Input: part model. Units: mm. Frame: model coordinates. A direction names the side the tool comes from. Give positions to 0.01 mm unless a question says otherwise; leave off trailing zeros. Order: outer loops, then holes, each group sorted by start corner. A loop starts at its lowest first (then second) coordinate and runs counter-clockwise, first axis right, second up. Notation, with made-up numbers: (-8.75, 57.25) - (7.25, 57.25) arc R23 cw to (7.25, 87.25) - close; hole circle Ø7 at (-5, 84.25). An arc over 180 degrees is marked (long way). Use a Markdown table: item, result.
from build123d import *

# Parameters (mm, degrees)
F0_W     = 19.05
F0_H     = 3.175
F1_DEPTH = 2.54


with BuildPart() as f1:
    # F0 (on Front) → F1 (new body)
    with BuildSketch(Plane.XZ):
        with BuildLine():
            Line((16.417073, 63.773632), (3.717073, 63.773632))
            Line((3.717073, 63.773632), (-8.982927, 63.773632))
            Line((-8.982927, 63.773632), (-8.982927, 69.615632))
            Line((-8.982927, 69.615632), (-37.430927, 69.615632))
            Line((-37.430927, 69.615632), (-37.430927, 41.834382))
            Line((-37.430927, 41.834382), (-34.382927, 41.834382))
            Line((-34.382927, 41.834382), (-34.382927, 14.053132))
            Line((-34.382927, 14.053132), (-37.430927, 14.053132))
            Line((-37.430927, 14.053132), (-37.430927, -13.728118))
            Line((-37.430927, -13.728118), (-34.382927, -13.728118))
            Line((-34.382927, -13.728118), (-34.382927, -41.509368))
            Line((-34.382927, -41.509368), (-28.032927, -41.509368))
            Line((-28.032927, -41.509368), (-28.032927, -35.159368))
            ThreePointArc((-28.032927, -35.159368), (-26.173055, -30.66924), (-21.682927, -28.809368))
            Line((-21.682927, -28.809368), (-19.142927, -28.809368))
            ThreePointArc((-19.142927, -28.809368), (-18.244901, -28.437393), (-17.872927, -27.539368))
            Line((-17.872927, -27.539368), (-17.872927, -24.364368))
            ThreePointArc((-17.872927, -24.364368), (-15.332927, -21.824368), (-12.792927, -24.364368))
            Line((-12.792927, -24.364368), (-12.792927, -27.539368))
            ThreePointArc((-12.792927, -27.539368), (-12.420952, -28.437393), (-11.522927, -28.809368))
            Line((-11.522927, -28.809368), (29.117073, -28.809368))
            ThreePointArc((29.117073, -28.809368), (33.607201, -30.66924), (35.467073, -35.159368))
            Line((35.467073, -35.159368), (35.467073, -41.509368))
            Line((35.467073, -41.509368), (44.865073, -41.509368))
            Line((44.865073, -41.509368), (44.865073, -13.728118))
            Line((44.865073, -13.728118), (41.817073, -13.728118))
            Line((41.817073, -13.728118), (41.817073, 14.053132))
            Line((41.817073, 14.053132), (44.865073, 14.053132))
            Line((44.865073, 14.053132), (44.865073, 41.834382))
            Line((44.865073, 41.834382), (41.817073, 41.834382))
            Line((41.817073, 41.834382), (41.817073, 69.615632))
            Line((41.817073, 69.615632), (16.417073, 69.615632))
            Line((16.417073, 69.615632), (16.417073, 63.773632))
        make_face()
        with Locations((3.717073, -17.696868)):
            Rectangle(F0_W, F0_H, mode=Mode.SUBTRACT)
    extrude(amount=F1_DEPTH)


solid = f1.part
1. Mould query, pull axis Z, two halves, no side actions, for faces 1 (the face through (4, -1, -16.109)), 2 (the face through (-20, -1, -28.809)), 3 (the face through (29, -1, 69.616)), 4 (the face through (16.417, -1, 67)). Classes: pulls with the +Z half, pulls with the -Z half, needs draft (parallel to the pull), parting line crosses it, or undercut.
Response:
| item | result |
|---|---|
| face 1 | undercut |
| face 2 | pulls with the -Z half |
| face 3 | pulls with the +Z half |
| face 4 | needs draft |
2. Section query A-A (x = 9). Return loops of the section in (y, z).
Response:
| item | result |
|---|---|
| outline | (-2.54, -28.81) - (0, -28.81) - (0, -19.28) - (-2.54, -19.28) - close; (-2.54, -16.11) - (0, -16.11) - (0, 63.77) - (-2.54, 63.77) - close |
3. Set-up query: faces 5 (the face through (33.56, -1.25, -30.62)), 6 (the face through (13.242, -1, -18)), 7 (the face through (-34.383, -1, 28)), 8 (the face through (-36, -1, -13.728)). Return all of +Z, -Z, +X, -X, +Y, -Y with unobstructed straight access to the full face (end or side cutting, diameter ignored); none if empty.
Response:
| item | result |
|---|---|
| face 5 | -Z, +Y, -Y |
| face 6 | +Y, -Y |
| face 7 | -X, +Y, -Y |
| face 8 | -Z, -X, +Y, -Y |
4. Material intervals for line 1 along Z through (x, y) = (3.5, -0.9); line 2 along X through (y, z) = (-1.6, -35); line 3 along X through (y, z) = (-2.2, -19.5), sorted ascending.
Response:
| item | result |
|---|---|
| line 1 | z = -28.81 to -19.28, -16.11 to 63.77 |
| line 2 | x = -34.38 to -28.03, 35.47 to 44.87 |
| line 3 | x = -34.38 to 44.87 |
5. Pin query (flat end, axial travel): pin 1 (0.8 mm diameter, centred on y = -1, z = -22.5, fed in from -X); pin 2 (0.8 mm diameter, centred on x = 43.5, y = -0.5, fed in from +Z); pin 3 (5 mm diameter, centred on x = 36.5, z = -4.5, fed in from +Y); pin 4 (0.8 mm diameter, centred on x = 7.5, y = -1.5, fed in from +Z). Return the tip coordinate at first contact, or that it passes through.
Response:
| item | result |
|---|---|
| pin 1 | stops at x = -34.38 |
| pin 2 | stops at z = 41.83 |
| pin 3 | stops at y = 0 |
| pin 4 | stops at z = 63.77 |
6. Section query B-B (z = -12). Return loops of the section in (x, y), then the cut area to 3 significant figures.
Response:
| item | result |
|---|---|
| outline | (-37.43, -2.54) - (41.82, -2.54) - (41.82, 0) - (-37.43, 0) - close |
| area | 201 mm^2 |
